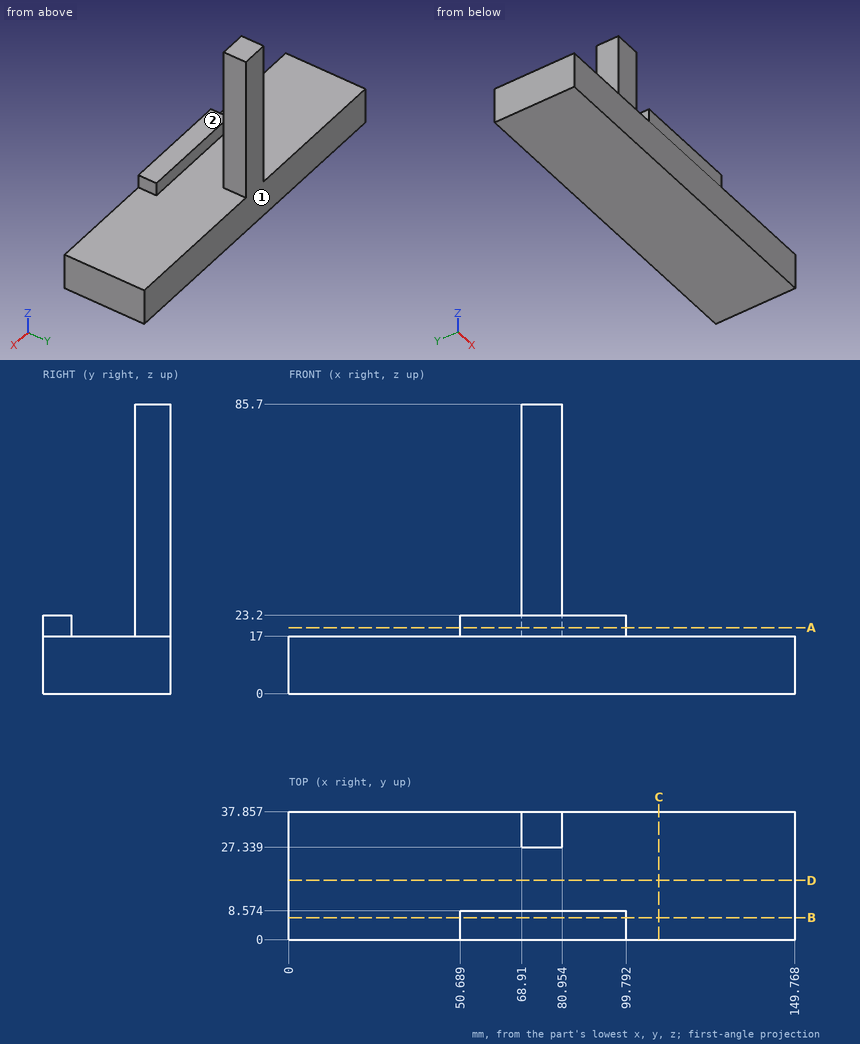
Answer from the drawing. Dimensions are ordinates in mm from the lowest x, y and z of the part. A direction names the side the tool comes from. Coordinates: 2 decimals unless noted, no trailing zeros. Loops run counter-clockwise (first coordinate to the right, second up) from the corner with the lowest first, then second, coordinate; pieces in that order, holes last. Notation, with made-up numbers: (-28, 83.25) - (29, 83.25) arc R12 cw to (29, 92.25) - close; hole circle Ø4 at (33.25, 44). An arc over 180 degrees is marked (long way). Answer in a Markdown table with one row per item.
1. Find section A-A, the plane z = 19.5. Write down the section's boundary in (x, y) (1 decimal).
Conclusion:
| item | result |
|---|---|
| outline | (50.7, 0) - (99.8, 0) - (99.8, 8.6) - (50.7, 8.6) - close; (68.9, 27.3) - (81, 27.3) - (81, 37.9) - (68.9, 37.9) - close |
2. Find section B-B, the plane y = 6.5. Write down the section's boundary in (x, z).
Conclusion:
| item | result |
|---|---|
| outline | (0, 0) - (149.77, 0) - (149.77, 17) - (99.79, 17) - (99.79, 23.2) - (50.69, 23.2) - (50.69, 17) - (0, 17) - close |
3. Straight lines are drawn through the part: line 1 (Z direction, x = 9.5, y = 11.5); line 2 (Y direction, x = 75, z = 30.5); line 3 (X direction, y = 4, z = 20). For each, find the intervals that lie inside material, in ascending order.
Conclusion:
| item | result |
|---|---|
| line 1 | z = 0 to 17 |
| line 2 | y = 27.34 to 37.86 |
| line 3 | x = 50.69 to 99.79 |
4. Given pin 1 (1.5 mm diameter, centred on x = 111.5, y = 32.5, fed in from +Z); pin 2 (10 mm diameter, centred on y = 25, z = 41.5, fed in from +X); pin 3 (7 mm diameter, centred on x = 76, y = 4.5, fed in from +Z); pin 4 (2 mm diameter, centred on x = 77.5, z = 9, fed in from -Y), each flat-ended and moving along its own axis, determine where each tip first touches the part or whether it passes through.
Conclusion:
| item | result |
|---|---|
| pin 1 | stops at z = 17 |
| pin 2 | stops at x = 80.95 |
| pin 3 | stops at z = 23.2 |
| pin 4 | stops at y = 0 |
5. Which of the six approach directions +Z, -Z, +X, -X, +Y, -Y give full straight-line access (tool end or side, diameter ignored) to the marked faces 1 and 2?
Conclusion:
| item | result |
|---|---|
| face 1 | +Z, -Z, +X, -X, +Y |
| face 2 | +Z, +X, -X, -Y |
6. Find section D-D, the plane y = 17.5. Write down the section's boundary in (x, z), then the cut area to 3 significant figures.
Conclusion:
| item | result |
|---|---|
| outline | (0, 0) - (149.77, 0) - (149.77, 17) - (0, 17) - close |
| area | 2,550 mm² |
7. Find section C-C, the plane x = 109.5. Write down the section's boundary in (y, z).
Conclusion:
| item | result |
|---|---|
| outline | (0, 0) - (37.86, 0) - (37.86, 17) - (0, 17) - close |
